For this review, take the finished solid that the model builds, in its own axes (mm). A direction names the side the tool comes from. Coordinates: 2 decimals unless noted, no trailing zeros. Loops run counter-clockwise (first coordinate to the right, second up) from the corner with the lowest first, then second, coordinate; pieces in that order, holes last. Notation, with made-up numbers: M -5.5,-2 L 17.5,-2 A27 cw 17.5,31 Z; hole C 61,-29.5 d8. An arc over 180 degrees is marked long. Use one line per item in the form item = value.
```python
from build123d import *

# Parameters (mm, degrees)
BOSS_EXTRUDE1_DEPTH = 15


with BuildPart() as part:
    # Sketch1 → Boss-Extrude1 (new body)
    with BuildSketch(Plane.XY):
        with BuildLine():
            Line((30.739596692, -3), (-30.739596692, -3))
            ThreePointArc((-30.739596692, -3), (-32.414147122, -3.288749544), (-33.895287282, -4.121647657))
            Line((-33.895287282, -4.121647657), (-48.34430941, -15.878352343))
            ThreePointArc((-48.34430941, -15.878352343), (-49.82544957, -16.711250456), (-51.5, -17))
            Line((-51.5, -17), (-56.5, -17))
            Line((-56.5, -17), (-56.5, -15))
            Line((-56.5, -15), (-51.5, -13))
            Line((-51.5, -13), (-51.5, -6.5))
            Line((-51.5, -6.5), (-56.5, -4.5))
            Line((-56.5, -4.5), (-56.5, -2.5))
            Line((-56.5, -2.5), (-38.387912283, -2.5))
            ThreePointArc((-38.387912283, -2.5), (-36.713361853, -2.211250456), (-35.232221692, -1.378352343))
            Line((-35.232221692, -1.378352343), (-34.916730933, -1.121647657))
            ThreePointArc((-34.916730933, -1.121647657), (-33.435590772, -0.288749544), (-31.761040342, 0))
            Line((-31.761040342, 0), (31.761040342, 0))
            ThreePointArc((31.761040342, 0), (33.435590772, -0.288749544), (34.916730933, -1.121647657))
            Line((34.916730933, -1.121647657), (35.232221692, -1.378352343))
            ThreePointArc((35.232221692, -1.378352343), (36.713361853, -2.211250456), (38.387912283, -2.5))
            Line((38.387912283, -2.5), (56.5, -2.5))
            Line((56.5, -2.5), (56.5, -4.5))
            Line((56.5, -4.5), (51.5, -6.5))
            Line((51.5, -6.5), (51.5, -13))
            Line((51.5, -13), (56.5, -15))
            Line((56.5, -15), (56.5, -17))
            Line((56.5, -17), (51.5, -17))
            ThreePointArc((51.5, -17), (49.82544957, -16.711250456), (48.34430941, -15.878352343))
            Line((48.34430941, -15.878352343), (33.895287282, -4.121647657))
            ThreePointArc((33.895287282, -4.121647657), (32.414147122, -3.288749544), (30.739596692, -3))
        make_face()
    extrude(amount=BOSS_EXTRUDE1_DEPTH)


solid = part.part
```
1. Tool access review of faces 1 (the face through (-48, -2.5, 7)), 2 (the face through (-49.803, -16.703, 7.395)), 3 (the face through (-54, -14, 7)), 4 (the face through (54, -5.5, 7.4)), 5 (the face through (47, -2.5, 7)): name each direction out of +Z, -Z, +X, -X, +Y, -Y from which nothing blocks a thin tool from reaching the whole face with its end or side.
Computed values:
face_1 = +Z, -Z, -X, +Y
face_2 = +Z, -Z, -Y
face_3 = +Z, -Z, -X
face_4 = +Z, -Z, +X
face_5 = +Z, -Z, +X, +Y
2. Draft analysis for pull direction X (two halves, no side actions). For faces 6 (the face through (-32.39, -3.28, 7.4)), 7 (the face through (54, -14, 7)), 8 (the face through (0.8, -2.7, 0)), state which applies: +X half, -X half, draft (parallel to the pull), parting line (faces both ways), or undercut.
Computed values:
face_6 = undercut
face_7 = +X half
face_8 = draft
3. Wall thickness on line 1 along Y through (x, z) = (-19.5, 6); line 2 along X through (y, z) = (-12, 10); line 3 along X through (y, z) = (-9, 3.5): over which ranges is each line inside the solid? List them lowest first. Write a range as from..to.
Computed values:
line_1 = -3..0
line_2 = -51.5..-43.58, 43.58..51.5
line_3 = -51.5..-39.89, 39.89..51.5
4. For pin 1 Ø4 at (x, z) = (19, 7.5) entering from -Y; pin 2 Ø1 at (x, z) = (-33.5, 1.5) entering from +Y; pin 3 Ø4.5 at (x, z) = (-46.5, 5) entering from +Y, all flat-tipped, find the tip position at first contact; note any pin that passes through.
Computed values:
pin_1 = -3
pin_2 = -0.16
pin_3 = -2.5
5. Consider section A-A on z = 2. Write out the cut boundary in (x, y), plus the area to 3 significant figures.
Computed values:
outline = M -56.5,-17 L -51.5,-17 A5 ccw -48.34,-15.88 L -33.9,-4.12 A5 cw -30.74,-3 L 30.74,-3 A5 cw 33.9,-4.12 L 48.34,-15.88 A5 ccw 51.5,-17 L 56.5,-17 L 56.5,-15 L 51.5,-13 L 51.5,-6.5 L 56.5,-4.5 L 56.5,-2.5 L 38.39,-2.5 A5 cw 35.23,-1.38 L 34.92,-1.12 A5 ccw 31.76,0 L -31.76,0 A5 ccw -34.92,-1.12 L -35.23,-1.38 A5 cw -38.39,-2.5 L -56.5,-2.5 L -56.5,-4.5 L -51.5,-6.5 L -51.5,-13 L -56.5,-15 Z
area = 578 mm2
6. Consider section B-B on y = -10. Write out the cut boundary in (x, z), plus the area to 3 significant figures.
Computed values:
outline = M -51.5,0 L -41.12,0 L -41.12,15 L -51.5,15 Z; M 41.12,0 L 51.5,0 L 51.5,15 L 41.12,15 Z
area = 311 mm2
7. Consider section D-D on y = -5.5. Write out the cut boundary in (x, z).
Computed values:
outline = M -54,0 L -35.59,0 L -35.59,15 L -54,15 Z; M 35.59,0 L 54,0 L 54,15 L 35.59,15 Z
8. Consider section C-C on x = 13. Write out the cut boundary in (y, z), plus the area to 3 significant figures.
Computed values:
outline = M -3,0 L 0,0 L 0,15 L -3,15 Z
area = 45.0 mm2
